Job drawing, mm, ordinate dimensions from the low corner. One solid piece. Give positions to 0.01 mm unless a question says otherwise; leave off trailing zeros. Order: outer loops, then holes, each group sorted by start corner. A loop starts at its lowest first (then second) coordinate and runs counter-clockwise, first axis right, second up.
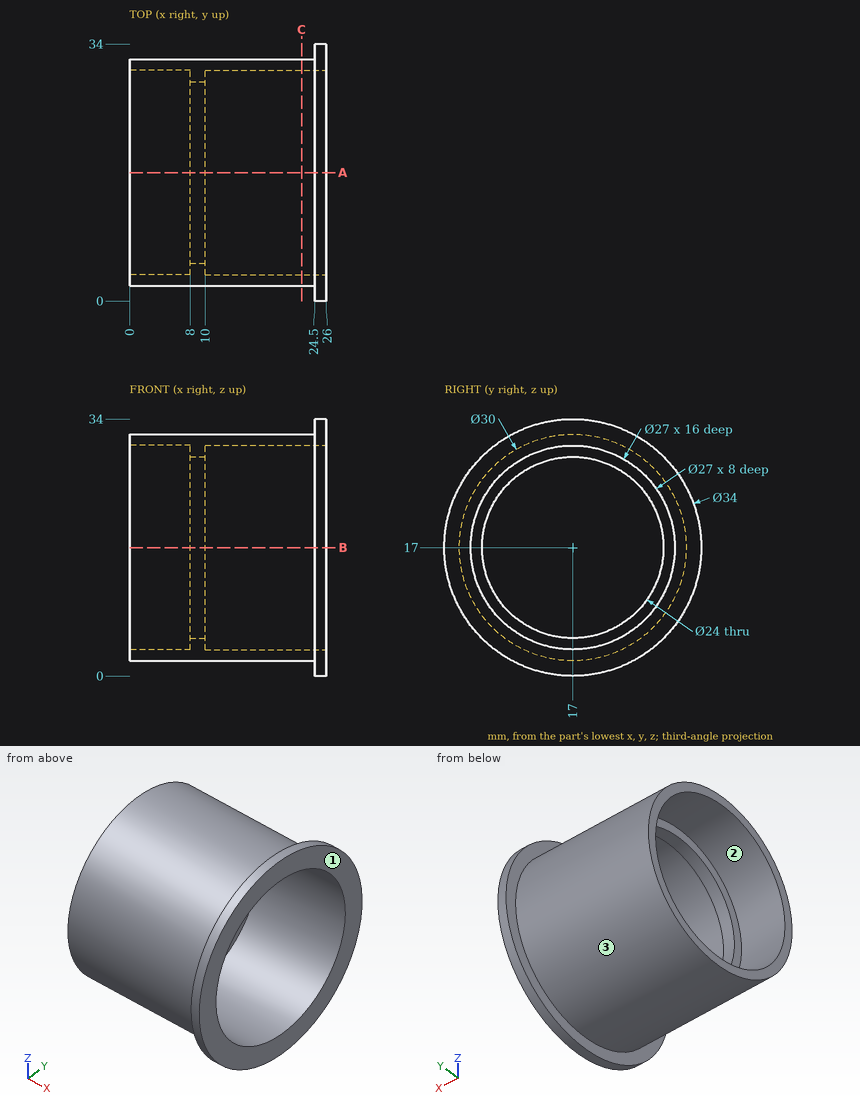
Item 1: Pull direction Z, two halves, no side cores. Call the marked faces 1, 2 and 3: released by +Z, released by -Z, zero draft, split by the parting line, or undercut.
Item 2: Drop flat-ended pins along their axis: P1, Ø2, axis at x = 22.5, y = 16.5, coming from the -Z side; P2, Ø12, axis at x = 19, z = 28, coming from the +Y side; P3, Ø5, axis at x = 13.5, z = 27.5, coming from the +Y side. Give the stop position or say it passes through.
Item 3: Band-saw the part on C-C on x = 22.75. List the corners of the cut face in (y, z), plus the area to 3 significant figures.
Item 4: Band-saw the part on A-A on y = 17. List the corners of the cut face in (x, z), plus the area to 3 significant figures.
Item 5: Drill centre lines: probe 1 along Y at (x, z) = (2.5, 17); probe 2 along Z at (x, y) = (9.05, 17). Where is each one in solid material? Low to high.
Working result:
1. face 1: zero draft
1. face 2: undercut
1. face 3: split by the parting line
2. P1: stops at z = 2
2. P2: stops at y = 31.66
2. P3: stops at y = 29.69
3. outline: circle Ø30 at (17, 17); hole circle Ø27 at (17, 17)
3. area: 134 mm2
4. outline: (0, 2) - (24.5, 2) - (24.5, 0) - (26, 0) - (26, 3.5) - (10, 3.5) - (10, 5) - (8, 5) - (8, 3.5) - (0, 3.5) - close; (0, 30.5) - (8, 30.5) - (8, 29) - (10, 29) - (10, 30.5) - (26, 30.5) - (26, 34) - (24.5, 34) - (24.5, 32) - (0, 32) - close
4. area: 90.0 mm2
5. probe 1: y = 2 to 3.5, 30.5 to 32
5. probe 2: z = 2 to 5, 29 to 32
